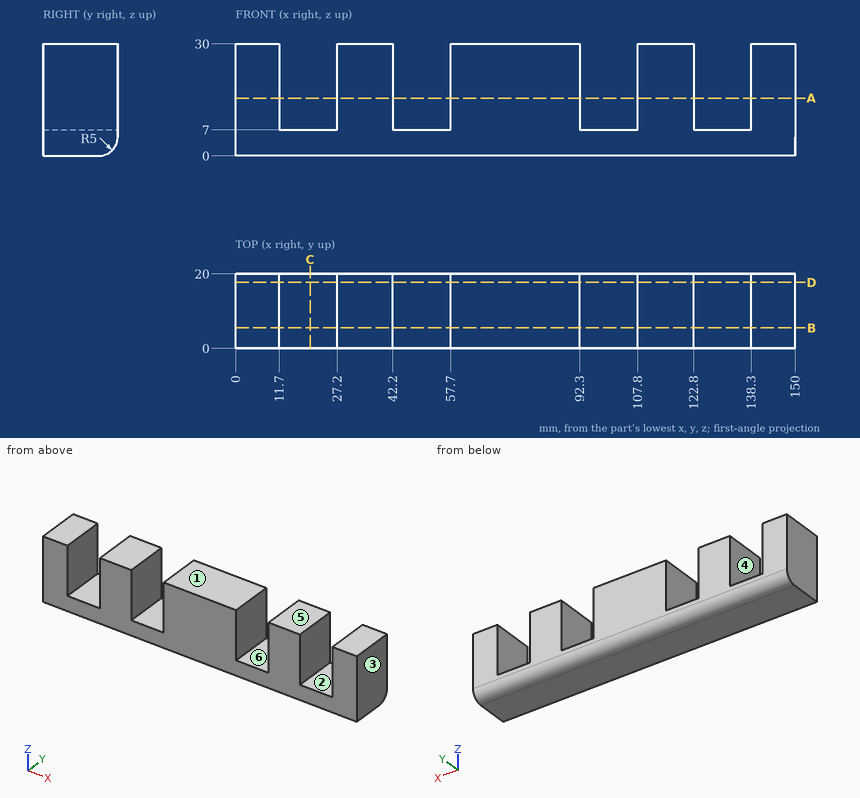
Geometry: see drawing. Coordinates: mm, zero at the bounding-box minimum. A direction names the side the tool comes from. Give positions to 0.01 mm unless a question says otherwise; leave off trailing zeros. Order: outer loops, then holes, each group sorted by start corner. A loop starts at its lowest first (then second) coordinate and runs counter-clockwise, first axis right, second up. Notation, with made-up numbers: (67, -1) -> (113, -1) arc R13 ccw to (113, 6) -> close; hole circle Ø8 at (-5, -37.75). An arc over 180 degrees is marked (long way). Write each question's results on one line, items separated by ' | '. Start each with the question number.
1) Section D-D (y = 17.75). Return loops of the section in (x, z), then the cut area to 3 significant figures.
2) Section C-C (x = 20). Return loops of the section in (y, z).
3) Section B-B (y = 5.5). Return loops of the section in (x, z).
4) Section A-A (z = 15.5). Return loops of the section in (x, y), then the cut area to 3 significant figures.
5) First-contact query: pin 1 (10 mm diameter, centred on y = 6.5, z = 22, fed in from -X); pin 2 (12 mm diameter, centred on x = 20.5, y = 10.5, fed in from +Z). Flat tips, straight axial feed; report the tip coordinate or a pass-through.
6) Line query: line 1 (X direction, y = 3, z = 17.25); line 2 (Z direction, x = 13.5, y = 12.5); line 3 (Y direction, x = 69, z = 4.5). Output: solid intervals per line, ascending. Write a range as from..to.
7) Set-up query: the marked faces 1 and 2. Return all of +Z, -Z, +X, -X, +Y, -Y with unobstructed straight access to the full face (end or side cutting, diameter ignored); none if empty.
8) Draft query along X for the marked faces 3, 4, 5 and 6. Return one class per face: pulls with the +X half, pulls with the -X half, needs draft (parallel to the pull), parting line crosses it, or undercut.
Calculated:
1) outline: (0, 0.82) -> (150, 0.82) -> (150, 30) -> (138.3, 30) -> (138.3, 7) -> (122.8, 7) -> (122.8, 30) -> (107.8, 30) -> (107.8, 7) -> (92.3, 7) -> (92.3, 30) -> (57.7, 30) -> (57.7, 7) -> (42.2, 7) -> (42.2, 30) -> (27.2, 30) -> (27.2, 7) -> (11.7, 7) -> (11.7, 30) -> (0, 30) -> close | area: 2,950 mm2
2) outline: (0, 0) -> (15, 0) arc R5 ccw to (20, 5) -> (20, 7) -> (0, 7) -> close
3) outline: (0, 0) -> (150, 0) -> (150, 30) -> (138.3, 30) -> (138.3, 7) -> (122.8, 7) -> (122.8, 30) -> (107.8, 30) -> (107.8, 7) -> (92.3, 7) -> (92.3, 30) -> (57.7, 30) -> (57.7, 7) -> (42.2, 7) -> (42.2, 30) -> (27.2, 30) -> (27.2, 7) -> (11.7, 7) -> (11.7, 30) -> (0, 30) -> close
4) outline: (0, 0) -> (11.7, 0) -> (11.7, 20) -> (0, 20) -> close; (27.2, 0) -> (42.2, 0) -> (42.2, 20) -> (27.2, 20) -> close; (57.7, 0) -> (92.3, 0) -> (92.3, 20) -> (57.7, 20) -> close; (107.8, 0) -> (122.8, 0) -> (122.8, 20) -> (107.8, 20) -> close; (138.3, 0) -> (150, 0) -> (150, 20) -> (138.3, 20) -> close | area: 1,760 mm2
5) pin 1: x = 0 | pin 2: z = 7
6) line 1: 0..11.7, 27.2..42.2, 57.7..92.3, 107.8..122.8, 138.3..150 | line 2: 0..7 | line 3: 0..19.97
7) face 1: +Z, +X, -X, +Y, -Y | face 2: +Z, +Y, -Y
8) face 3: pulls with the +X half | face 4: undercut | face 5: needs draft | face 6: undercut
